Input: part model. Units: mm. Frame: model coordinates. Face numbers are marked on the shaded views. Coordinates: 2 decimals unless noted, no trailing zeros.
(1) Line query: L1, parallel to Y at x = 7.5, z = -23; L2, parallel to Z at x = 4.25, y = -11.5; L3, parallel to Y at x = 3.75, z = 31. Output: solid intervals per line, ascending.
(2) Mould query, pull axis Z, two halves, no side actions, for the marked faces 1, 2 and 3. Classes: released by +Z, released by -Z, zero draft, split by the parting line, or undercut.
(3) Contact query for flat-ended pins moving along their axis: P1, Ø3.5, axis at y = 7.39, z = -25.56, coming from the +X side; P2, Ø5, axis at y = 2.39, z = 44.44, coming from the -X side. Output: stop coordinate, or through.
(4) Section A-A, the plane x = 4.5. Give the number of separate pieces and of enclosed holes in the cut face, then the cut area to 3 significant figures.
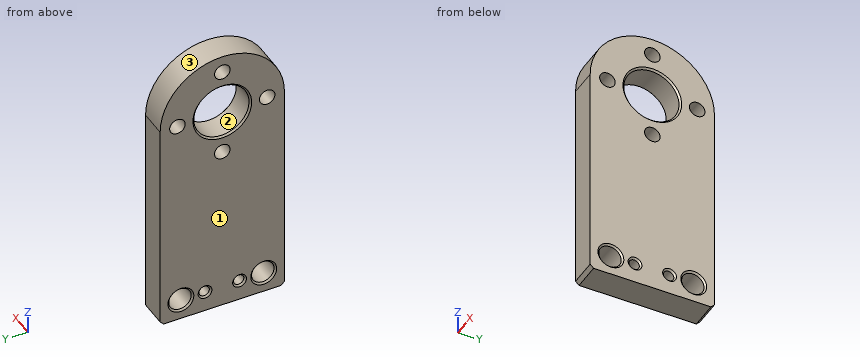
```python
from build123d import *

# Parameters (mm, degrees)
SKETCH1_R           = 8
SKETCH1_R_2         = 2.25
SKETCH1_R_3         = 3.25
SKETCH1_R_4         = 1.5
BOSS_EXTRUDE1_DEPTH = 8
CHAMFER1_SIZE       = 1
CHAMFER2_SIZE       = 0.5


with BuildPart() as part:
    # Sketch1 → Boss-Extrude1 (new body)
    with BuildSketch(Plane(origin=(0, 0, 0), x_dir=(0, 0, -1), z_dir=(1, 0, 0))):
        with BuildLine():
            Line((-31.438596491, 20.385964912), (31.561403509, 20.385964912))
            Line((31.561403509, 20.385964912), (31.561403509, -15.614035088))
            Line((31.561403509, -15.614035088), (-31.438596491, -15.614035088))
            ThreePointArc((-31.438596491, -15.614035088), (-49.438596491, 2.385964912), (-31.438596491, 20.385964912))
        make_face()
        with Locations((-31.438596491, 2.385964912)):
            Circle(SKETCH1_R, mode=Mode.SUBTRACT)
        with Locations((-31.438596491, 15.385964912)):
            Circle(SKETCH1_R_2, mode=Mode.SUBTRACT)
        with Locations((-18.438596491, 2.385964912)):
            Circle(SKETCH1_R_2, mode=Mode.SUBTRACT)
        with Locations((-31.438596491, -10.614035088)):
            Circle(SKETCH1_R_2, mode=Mode.SUBTRACT)
        with Locations((-44.438596491, 2.385964912)):
            Circle(SKETCH1_R_2, mode=Mode.SUBTRACT)
        with Locations((25.561403509, 14.385964912)):
            Circle(SKETCH1_R_3, mode=Mode.SUBTRACT)
        with Locations((25.561403509, 7.385964912)):
            Circle(SKETCH1_R_4, mode=Mode.SUBTRACT)
        with Locations(Location((25.561403509, -2.614035088, 0), (0, 0, 180))):
            Circle(SKETCH1_R_4, mode=Mode.SUBTRACT)
        with Locations(Location((25.561403509, -9.614035088, 0), (0, 0, 180))):
            Circle(SKETCH1_R_3, mode=Mode.SUBTRACT)
    extrude(amount=BOSS_EXTRUDE1_DEPTH)

    # Chamfer1
    chamfer1_edges = [part.edges().sort_by_distance(p)[0] for p in [
        (4, 20.385964912, -31.561403509),
        (4, -15.614035088, -31.561403509),
    ]]
    chamfer(chamfer1_edges, length=CHAMFER1_SIZE)

    # Chamfer2
    chamfer2_edges = [part.edges().sort_by_distance(p)[0] for p in [
        (0, 2.385964912, 39.438596491),
        (8, 2.385964912, 39.438596491),
        (0, 14.385964912, -22.311403509),
        (8, 14.385964912, -22.311403509),
        (0, 7.385964912, -24.061403509),
        (8, 7.385964912, -24.061403509),
        (0, -2.614035088, -27.061403509),
        (8, -2.614035088, -27.061403509),
        (0, -9.614035088, -28.811403509),
        (8, -9.614035088, -28.811403509),
    ]]
    chamfer(chamfer2_edges, length=CHAMFER2_SIZE)


solid = part.part
```
Report:
1. L1: y = -15.61 to -11.61, -7.61 to 12.39, 16.39 to 20.39
1. L2: z = -31.56 to -28.21, -22.91 to 29.37, 33.51 to 42.89
1. L3: y = -15.61 to -12.82, -8.41 to -5.6, 10.37 to 13.18, 17.59 to 20.39
2. face 1: zero draft
2. face 2: undercut
2. face 3: released by +Z
3. P1: stops at x = 7.75
3. P2: stops at x = 0
4. separate pieces: 1
4. enclosed holes: 9
4. area: 2,430 mm2
